Geometry: final body of the model. Coordinates: model frame, mm. A direction names the side the tool comes from. Give positions to 0.01 mm unless a question says otherwise; leave off trailing zeros. Write each loop counter-clockwise with the first axis right and the second up, starting at its lowest first coordinate (ties: lowest second). Pieces come first, ordered by that corner, then holes. Notation, with made-up numbers: M 3.25,-13.5 L 10.25,-13.5 A28 cw 10.25,18.5 Z; hole C 0.5,-15 d4. An arc over 180 degrees is marked long. Use a Markdown table: item, result. Add a question column.
(1) Cut plane B-B (z = -0.7). Output: boundary loops of the cut face in (x, y).
(2) Draft query along Y for faces 1 (the flat face through (100, 25, -1)), 2 (the flat face through (4.8, 12, -1)). Return one class per face: released by +Y, released by -Y, zero draft, split by the parting line, or undercut.
(3) Cut plane A-A (y = 38). Output: boundary loops of the cut face in (x, z), plus the area to 3 significant figures.
(4) Reachability of faces 3 (the flat face through (97, 31.6, -1)), 4 (the flat face through (49, 25, 0)) from +Z, -Z, +X, -X, +Y, -Y: full face, straight path, thin tool, end or side. Return the list, or none.
(5) Material intervals for L1, parallel to X at y = 11.5, z = -1.6, sorted ascending.
```python
from build123d import *

# Parameters (mm, degrees)
SKETCH_1_W      = 100
SKETCH_1_H      = 50
SKETCH_1_W_2    = 2.8
SKETCH_1_H_2    = 11.8
EXTRUDE_1_DEPTH = 3


with BuildPart() as part:
    # Эскиз1 → Бобышка-Вытянуть1 (new body)
    with BuildSketch(Plane.XY):
        with Locations((50, 25)):
            Rectangle(SKETCH_1_W, SKETCH_1_H)
        with Locations((3.4, 37.5)):
            Rectangle(SKETCH_1_W_2, SKETCH_1_H_2, mode=Mode.SUBTRACT)
        with Locations((3.4, 12.5)):
            Rectangle(SKETCH_1_W_2, SKETCH_1_H_2, mode=Mode.SUBTRACT)
        with Locations((96.6, 12.5)):
            Rectangle(SKETCH_1_W_2, SKETCH_1_H_2, mode=Mode.SUBTRACT)
        with Locations((96.6, 37.5)):
            Rectangle(SKETCH_1_W_2, SKETCH_1_H_2, mode=Mode.SUBTRACT)
    extrude(amount=-EXTRUDE_1_DEPTH)


solid = part.part
```
Answer list:
| question | item | result |
|---|---|---|
| 1 | outline | M 0,0 L 100,0 L 100,50 L 0,50 Z; hole M 2,6.6 L 4.8,6.6 L 4.8,18.4 L 2,18.4 Z; hole M 2,31.6 L 4.8,31.6 L 4.8,43.4 L 2,43.4 Z; hole M 95.2,6.6 L 98,6.6 L 98,18.4 L 95.2,18.4 Z; hole M 95.2,31.6 L 98,31.6 L 98,43.4 L 95.2,43.4 Z |
| 2 | face 1 | zero draft |
| 2 | face 2 | undercut |
| 3 | outline | M 0,-3 L 2,-3 L 2,0 L 0,0 Z; M 4.8,-3 L 95.2,-3 L 95.2,0 L 4.8,0 Z; M 98,-3 L 100,-3 L 100,0 L 98,0 Z |
| 3 | area | 283 mm² |
| 4 | face 3 | +Z, -Z |
| 4 | face 4 | +Z, +X, -X, +Y, -Y |
| 5 | L1 | 0 to 2, 4.8 to 95.2, 98 to 100 |
